CAD build for the part. Positions are in the model's coordinates, mm. A direction names the side the tool comes from. Round coordinates to 2 decimals unless told otherwise and drop trailing zeros. Loops run counter-clockwise (first coordinate to the right, second up) from the corner with the lowest first, then second, coordinate; pieces in that order, holes last.
Autodesk Inventor part; units mm, degrees
ref_plane "YZ Plane" through (0, 0, 0) normal (1, 0, 0) x (0, 1, 0)
ref_plane "XZ Plane" through (0, 0, 0) normal (0, 1, 0) x (-1, 0, 0)
ref_plane "XY Plane" through (0, 0, 0) normal (0, 0, 1) x (1, 0, 0)
sketch "Szkic1" plane through (0, 0, 0) normal (0, 1, 0) x (-1, 0, 0)
  line L0 (25, 19) -> (-25, 19)
  line L1 (-25, 19) -> (-25, -19)
  line L2 (-25, -19) -> (25, -19)
  line L3 (25, -19) -> (25, 19)
  line L4 (25, 19) -> (-25, -19) construction
  line L5 (-25, 19) -> (25, -19) construction
  point P0 (0, 0)
  dimension "d0" = 50
  dimension "d1" = 38
extrude "Wyciągnięcie proste1" add sketch "Szkic1" along normal blind 4
sketch "Szkic2" plane through (0, 4, 0) normal (0, 1, 0) x (1, 0, 0)
  line L0 (-25, 19) -> (-25, -19)
  line L1 (25, -19) -> (25, 19)
  line L2 (-25, 19) -> (25, 19)
  line L3 (25, 19) -> (25, 15)
  line L4 (25, 15) -> (-25, 15)
  line L5 (-25, 15) -> (-25, 19)
  point P0 (0, 0)
  dimension "d4" = 4
extrude "Wyciągnięcie proste2" add sketch "Szkic2" along normal blind 34
sketch "Szkic3" plane through (0, 4, 0) normal (0, 1, 0) x (1, 0, 0)
  line L0 (25, -19) -> (25, 19)
  line L1 (25, 0) -> (-25, 0) construction
  line L2 (-25, 19) -> (-25, -19)
  line L3 (-25, 15) -> (25, 15)
  line L4 (0, 15) -> (0, -19) construction
  line L5 (0, -15) -> (0, 19) construction
  point P0 (0, 0)
  point P1 (-11, 8)
  point P2 (-11, -8)
  point P3 (11, 8)
  point P4 (11, -8)
  dimension "d7" = 8
  dimension "d8" = 11
hole "Otwór1" at (-11, 4, -8) at (-11, 4, 8) at (11, 4, 8) at (11, 4, -8) direction (0, -1, 0) diameter 3 depth 8 tip angle 118
sketch "Szkic4" plane through (-25, 4, -15) normal (0, 0, 1) x (1, 0, 0)
  line L0 (50, 34) -> (0, 34)
  line L1 (0, 0) -> (0, 34)
  line L2 (50, 0) -> (0, 0)
  line L3 (25, 34) -> (25, 0) construction
  point P0 (25, -4)
  point P1 (25, 26)
  point P2 (13, 10)
  point P3 (37, 10)
  dimension "d16" = 8
  dimension "d17" = 25
  dimension "d18" = 13
  dimension "d19" = 10
hole "Otwór2" at (0, 30, -15) at (-12, 14, -15) at (12, 14, -15) direction (0, 0, -1) diameter 3 depth 8 tip angle 118
sketch "Szkic5" plane through (-25, 4, -15) normal (0, 0, 1) x (1, 0, 0)
  line L0 (0, 34) -> (50, 34)
  line L1 (50, 0) -> (50, 34)
  line L2 (50, 0) -> (0, 0)
  line L3 (34, 34) -> (50, 0)
  line L4 (34, 34) -> (50, 34)
  line L5 (50, 34) -> (50, 0)
  line L6 (25, 34) -> (25, 0) construction
  line L7 (50, 34) -> (0, 34)
  line L8 (0, 0) -> (0, 34)
  line L9 (0, 0) -> (50, 0)
  line L10 (16, 34) -> (0, 0)
  line L11 (16, 34) -> (0, 34)
  line L12 (0, 34) -> (0, 0)
  point P0 (25, -4)
  dimension "d27" = 16
extrude "Wyciągnięcie proste3" cut sketch "Szkic5" against normal blind 34 contours L0 L10 L8 | L0 L1 L3
fillet "Zaokrąglenie1" radius 4 2 edges at (-9, 38, -17) (9, 38, -17)
sketch "Szkic7" plane through (0, 4, 0) normal (0, 1, 0) x (1, 0, 0)
  line L0 (25, 15) -> (-25, 15)
  line L1 (-2, 15) -> (2, 15)
  line L2 (2, 15) -> (2, -5)
  line L3 (2, -5) -> (-2, -5)
  line L4 (-2, -5) -> (-2, 15)
  point P0 (0, 0)
  dimension "d31" = 4
  dimension "d32" = 20
  dimension "d33" = 2
extrude "Wyciągnięcie proste4" add sketch "Szkic7" along normal blind 20
sketch "Szkic8" plane through (2, 4, 5) normal (1, 0, 0) x (0, 0, -1)
  line L0 (20, 20) -> (0, 20)
  line L1 (20, 20) -> (0, 0)
  line L2 (0, 0) -> (0, 20)
  line L3 (-14, -4) -> (24, -4)
  line L4 (0, 20) -> (20, 20)
  point P0 (5, -4)
extrude "Wyciągnięcie proste5" cut sketch "Szkic8" against normal blind 18
sketch "Szkic9" plane through (25, 0, 19) normal (1, 0, 0) x (0, 0, -1)
  line L0 (38, 0) -> (0, 0)
  line L1 (38, 0) -> (37, 0)
  line L2 (37, 0) -> (37, 38)
  line L3 (37, 38) -> (38, 38)
  line L4 (38, 38) -> (38, 0)
  point P0 (19, 0)
  dimension "d38" = 1
  dimension "d39" = 38
extrude "Wyciągnięcie proste6" cut sketch "Szkic9" against normal through all
chamfer "Faza1" distance 15 angle 45 2 edges at (25, 2, 19) (-25, 2, 19)
fillet "Zaokrąglenie2" radius 10 4 edges at (25, 2, 4) (10, 2, 19) (-10, 2, 19) (-25, 2, 4)
properties part number "Wspornik" material "Tworzywo sztuczne PET"
Item 1: Cut at C-C (y = 30). List the corners of the cut face in (x, z).
Verdict:
outline: (-12.76, -18) - (-1.5, -18) - (-1.5, -15) - (-12.76, -15) - close; (1.5, -18) - (12.76, -18) - (12.76, -15) - (1.5, -15) - close
Item 2: Cut at D-D (z = -12.5). List the corners of the cut face in (x, y).
Verdict:
outline: (-25, 0) - (25, 0) - (25, 4) - (2, 4) - (2, 21.5) - (-2, 21.5) - (-2, 4) - (-25, 4) - close
Item 3: 3-axis set-ups, long thin cutter, end or side, ignore diameter. For faces 5 (the flat face through (2, 12, -7)), 6 (the flat face through (0, 4, 6)), 7 (the cylindrical face through (-8.63, 37.36, -16.52)): which of +Z, -Z, +X, -X, +Y, -Y reach the whole face in a straight line?
Verdict:
face 5: +Z, +X, +Y
face 6: +Z, +Y
face 7: +Z, -Z, -X, +Y
Item 4: Cut at B-B (z = 8). List the corners of the cut face in (x, y).
Verdict:
outline: (-21, 0) - (-12.5, 0) - (-12.5, 4) - (-21, 4) - close; (-9.5, 0) - (9.5, 0) - (9.5, 4) - (-9.5, 4) - close; (12.5, 0) - (21, 0) - (21, 4) - (12.5, 4) - close
Item 5: Flat gauge pins, fed straight in: P1, Ø4, axis at y = 18.5, z = -9, coming from the +X side; P2, Ø1.5, axis at x = -3, z = 2, coming from the +Y side; P3, Ø16, axis at y = 12.5, z = -9, coming from the -X side; P4, Ø2.5, axis at x = -11, z = 8, coming from the -Y side. Where does each tip first touch, or does it go through?
Verdict:
P1: stops at x = 2
P2: stops at y = 4
P3: stops at x = -23.49
P4: passes through
Item 6: Wall check: L1, parallel to X at y = 2, z = -8; L2, parallel to X at y = 14, z = -16.3; L3, parallel to Y at x = 0, z = -16.95. Give the ranges that are in metal, low to high.
Verdict:
L1: x = -25 to -12.5, -9.5 to 9.5, 12.5 to 25
L2: x = -20.29 to -13.5, -10.5 to 10.5, 13.5 to 20.29
L3: y = 0 to 28.5, 31.5 to 38
Item 7: Cut at A-A (x = 0). List the corners of the cut face in (y, z).
Verdict:
outline: (0, -18) - (28.5, -18) - (28.5, -15) - (24, -15) - (4, 5) - (4, 19) - (0, 19) - close; (31.5, -18) - (38, -18) - (38, -15) - (31.5, -15) - close
Item 8: Mould opens along Z. For faces 1 (the cylindrical face through (-10.1, 2, 6.8)), 2 (the flat face through (0, 15, -18)), 3 (the cylindrical face through (11.9, 2, 6.8)), 4 (the flat face through (-2, 9, -9)) say: released by +Z, released by -Z, zero draft, split by the parting line, or undercut.
Verdict:
face 1: undercut
face 2: released by -Z
face 3: undercut
face 4: zero draft
